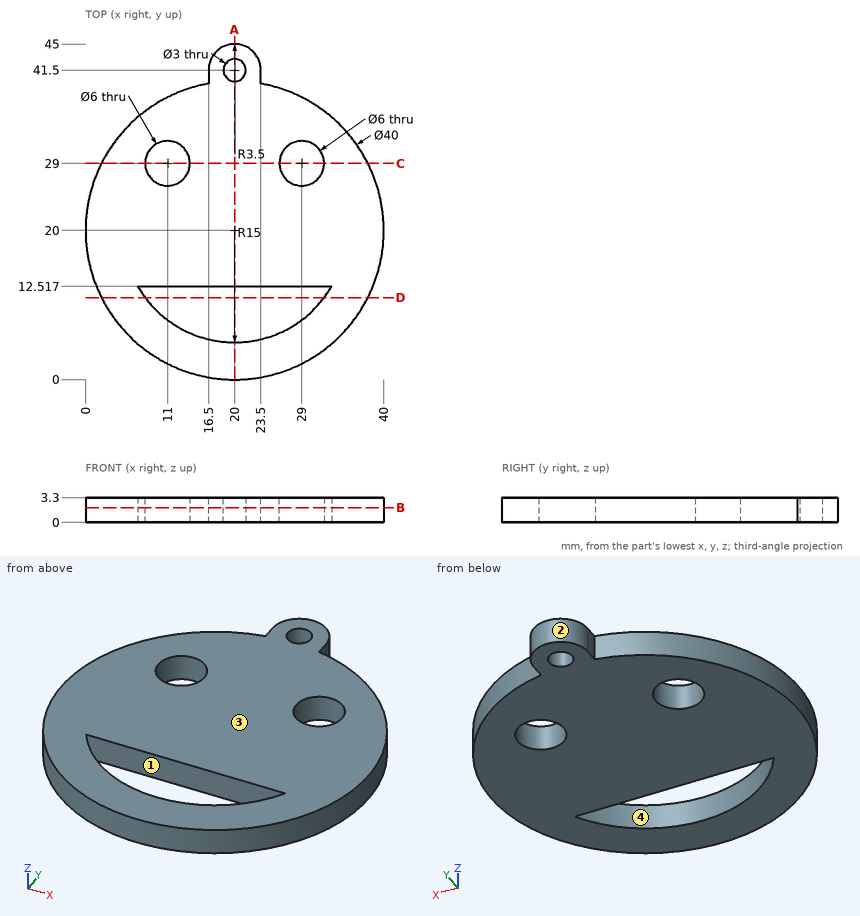
Study the drawing (mm; zero at the part's minimum x, y, z) and answer. Give positions to 0.01 mm unless a question says otherwise; leave off trailing zeros. Write each loop counter-clockwise with the first axis right and the second up, starting at its lowest first coordinate (ties: lowest second). Pieces come first, ordered by that corner, then holes. Notation, with made-up numbers: M -34.75,58.5 L 1.25,58.5 A10 ccw 1.25,67.5 Z; hole C 74,-38.75 d1. An arc over 180 degrees is marked long. Put each result on its own line as item: value. Start each with the question number.
1. For a pull along X with two mould halves and no side action, classify the marked faces 1, 2, 3 and 4 as released by +X, released by -X, zero draft, split by the parting line, or undercut.
2. The part is cut by section C-C, the plane y = 29. Give the vertices of the cut face in (x, z).
3. The part is cut by section B-B, the plane z = 1.95. Give the vertices of the cut face in (x, y), and give its area (4 significant figures).
4. The part is cut by section D-D, the plane y = 11. Give the vertices of the cut face in (x, z).
5. Each of these flat-tipped pins is pushed along its axis until it touches: pin 1 Ø0.5 at (y, z) = (40.5, 1.5) entering from -X; pin 2 Ø1 at (x, z) = (26.5, 1) entering from -Y. Where does it stop, or does it pass through?
6. The part is cut by section A-A, the plane x = 20. Give the vertices of the cut face in (y, z).
7. Consider line 1 along Y through (x, z) = (26.5, 1.45) (1 decimal); line 2 along Y through (x, z) = (12, 2.2); line 3 along X through (y, z) = (28.5, 3.15) (1 decimal). Determine where each line is inside the solid, lowest interval first.
Final values:
1. face 1: undercut
1. face 2: split by the parting line
1. face 3: zero draft
1. face 4: undercut
2. outline: M 2.14,0 L 8,0 L 8,3.3 L 2.14,3.3 Z; M 14,0 L 26,0 L 26,3.3 L 14,3.3 Z; M 32,0 L 37.86,0 L 37.86,3.3 L 32,3.3 Z
3. outline: M 16.5,39.69 A20 ccw long 23.5,39.69 L 23.5,41.5 A3.5 ccw 16.5,41.5 Z; hole M 7,12.52 A15 ccw 33,12.52 Z; hole C 11,29 d6; hole C 20,41.5 d3; hole C 29,29 d6
3. area: 1,085 mm²
4. outline: M 2.14,0 L 8,0 L 8,3.3 L 2.14,3.3 Z; M 32,0 L 37.86,0 L 37.86,3.3 L 32,3.3 Z
5. pin 1: stops at x = 16.5
5. pin 2: stops at y = 0.92
6. outline: M 0,0 L 5,0 L 5,3.3 L 0,3.3 Z; M 12.52,0 L 40,0 L 40,3.3 L 12.52,3.3 Z; M 43,0 L 45,0 L 45,3.3 L 43,3.3 Z
7. line 1: y = 1.1 to 6.5, 12.5 to 27.3, 30.7 to 38.9
7. line 2: y = 1.67 to 7.31, 12.52 to 26.17, 31.83 to 38.33
7. line 3: x = 1.9 to 8, 14 to 26, 32 to 38.1
